```python
from build123d import *

# Parameters (mm, degrees)
F0_W      = 21.620078
F0_H      = 30.16656
F0_W_2    = 19.802009
F0_W_3    = 35.716062
F1_DEPTH  = 25
F2_W      = 85.43355
F2_H      = 25
F3_DEPTH  = 5
F4_W      = 85.43355
F4_H      = 25
F5_DEPTH  = 5
F6_W      = 30.16656
F6_H      = 25
F7_DEPTH  = 5
F8_W      = 30.16656
F8_H      = 25
F9_DEPTH  = 5
F11_DEPTH = 5


with BuildPart() as f1:
    # F0 (on Top) → F1 (new body)
    with BuildSketch(Plane.XY):
        Polygon((-36.758605, 15.372929), (-38.758605, 13.372929), (-38.758605, -16.793631), (-36.758605, -18.793631), (48.674945, -18.793631), (50.674945, -16.793631), (50.674945, 13.372929), (48.674945, 15.372929), align=None)
        with Locations((-25.948566, -1.710351)):
            Rectangle(F0_W, F0_H, mode=Mode.SUBTRACT)
        with Locations((-1.321006, -1.710351)):
            Rectangle(F0_W_2, F0_H, mode=Mode.SUBTRACT)
        with Locations((30.816914, -1.710351)):
            Rectangle(F0_W_3, F0_H, mode=Mode.SUBTRACT)
    extrude(amount=F1_DEPTH)

    # F2 (on face) → F3 (join)
    with BuildSketch(Plane(origin=(0, 15.372929, 0), x_dir=(-1, 0, 0), z_dir=(0, 1, 0))):
        with Locations((-5.95817, 12.5)):
            Rectangle(F2_W, F2_H)
    extrude(amount=F3_DEPTH)

    # F4 (on face) → F5 (join)
    with BuildSketch(Plane.XZ.offset(18.793631)):
        with Locations((5.95817, 12.5)):
            Rectangle(F4_W, F4_H)
    extrude(amount=F5_DEPTH)

    # F6 (on face) → F7 (join)
    with BuildSketch(Plane(origin=(-38.758605, 0, 0), x_dir=(0, -1, 0), z_dir=(-1, 0, 0))):
        with Locations((1.710351, 12.5)):
            Rectangle(F6_W, F6_H)
    extrude(amount=F7_DEPTH)

    # F8 (on face) → F9 (join)
    with BuildSketch(Plane.YZ.offset(50.674945)):
        with Locations((-1.710351, 12.5)):
            Rectangle(F8_W, F8_H)
    extrude(amount=F9_DEPTH)

    # F10 (on face) → F11 (join)
    with BuildSketch(Plane(origin=(0, 20.372929, 0), x_dir=(-1, 0, 0), z_dir=(0, 1, 0))):
        Polygon((36.758605, 25), (-48.674945, 0), (36.758605, 0), align=None)
    extrude(amount=F11_DEPTH)


solid = f1.part
```
Can you work these out from the model? Positions are in its coordinate system, mm. A direction names the side the tool comes from. Round coordinates to 2 decimals unless told otherwise and drop trailing zeros. Loops run counter-clockwise (first coordinate to the right, second up) from the corner with the lowest first, then second, coordinate; pieces in that order, holes last.
Item 1: If we mould it in two halves opening along Y, with no side actions, what happens to faces 4 (the flat face through (-15.139, -2, 12)), 5 (the flat face through (55.675, -2, 13)), 6 (the flat face through (53, -16.794, 12))? For each: +Y half, -Y half, draft (parallel to the pull), parting line (faces both ways), or undercut.
Item 2: Suppose I cut it at D-D, the plane x = -14. Write out the boundary of the cut face in (y, z).
Item 3: Suppose I cut it at C-C, the plane z = 6.5. State how many separate pieces and enclosed holes the cut face has, then the cut area to 3 significant figures.
Item 4: Which directions (+Z, -Z, +X, -X, +Y, -Y) give clear straight access to the entire face, cutting with the end or side of a thin tool? Please do faces 1 (the flat face through (8.58, -2, 12)), 2 (the flat face through (-41, -16.794, 12)), 3 (the flat face through (16, 20.373, 15)).
Item 5: Please list where these lines run through material, in increasing order: L1, parallel to X at y = 1, z = 19.5; L2, parallel to Y at x = -21.5, z = 16; L3, parallel to Y at x = 22, z = 20.25.
Item 6: Suppose I cut it at B-B, the plane x = 41. Write out the boundary of the cut face in (y, z).
Item 7: Will these pins go through, and if not, where does the flat tip stop? pin 1 Ø2 at (x, z) = (14, 22) entering from +Y; pin 2 Ø4 at (y, z) = (-20.5, 14.5) entering from +X; pin 3 Ø4 at (y, z) = (17, 14) entering from -X.
Item 8: Suppose I cut it at A-A, the plane y = -2.5. Write out the boundary of the cut face in (x, z), then the cut area to 3 significant figures.
Reported:
1. face 4: undercut
1. face 5: draft
1. face 6: -Y half
2. outline: (-23.79, 0) - (25.37, 0) - (25.37, 18.34) - (20.37, 18.34) - (20.37, 25) - (-23.79, 25) - close
3. separate pieces: 1
3. enclosed holes: 3
3. area: 2,190 mm2
4. face 1: +Z, -Z
4. face 2: +Z, -Z, -X, -Y
4. face 3: +Z, +X, +Y
5. L1: x = -43.76 to -36.76, -15.14 to -11.22, 8.58 to 12.96, 48.67 to 55.67
5. L2: y = -23.79 to -16.79, 13.37 to 25.37
5. L3: y = -23.79 to -16.79, 13.37 to 20.37
6. outline: (-23.79, 0) - (-16.79, 0) - (-16.79, 25) - (-23.79, 25) - close; (13.37, 0) - (25.37, 0) - (25.37, 2.25) - (20.37, 2.25) - (20.37, 25) - (13.37, 25) - close
7. pin 1: stops at y = 20.37
7. pin 2: stops at x = 48.97
7. pin 3: stops at x = -37.13
8. outline: (-43.76, 0) - (-36.76, 0) - (-36.76, 25) - (-43.76, 25) - close; (-15.14, 0) - (-11.22, 0) - (-11.22, 25) - (-15.14, 25) - close; (8.58, 0) - (12.96, 0) - (12.96, 25) - (8.58, 25) - close; (48.67, 0) - (55.67, 0) - (55.67, 25) - (48.67, 25) - close
8. area: 557 mm2
